Autodesk Inventor part; units mm, degrees
ref_plane "YZ Plane" through (0, 0, 0) normal (1, 0, 0) x (0, 1, 0)
ref_plane "XZ Plane" through (0, 0, 0) normal (0, 1, 0) x (-1, 0, 0)
ref_plane "XY Plane" through (0, 0, 0) normal (0, 0, 1) x (1, 0, 0)
sketch "Sketch1" plane through (0, 0, 0) normal (0, 1, 0) x (-1, 0, 0)
  circle A0 centre (0, 0) radius 6.325
  circle A1 centre (-118.053, 0) radius 6.325
  circle A2 centre (-74.04, -14.35) radius 4.5
  circle A3 centre (-74.04, 14.35) radius 4.5
  circle A4 centre (-105.29, 19.35) radius 4.5
  line L0 (-4.4447, 4.5) -> (-9.5157, 4.5)
  line L1 (-9.5157, 4.5) -> (-73.0558, 18.7411)
  line L2 (-73.329, 18.7935) -> (-104.579, 23.7935)
  line L3 (-119.775, -6.0861) -> (-75.2652, -18.68)
  line L4 (-75.2652, 18.68) -> (-119.775, 6.0861)
  line L5 (-109.79, 19.35) -> (-109.79, 8.9113)
  line L6 (-69.54, 14.35) -> (-69.54, -14.35)
  line L7 (-78.54, 14.35) -> (-78.54, -14.35)
  line L8 (-108.8889, 0) -> (-78.54, 8.5871)
  line L9 (-108.8889, 0) -> (-78.54, -8.5871)
  line L10 (-4.4447, -4.5) -> (-9.5157, -4.5)
  line L11 (-9.5157, -4.5) -> (-73.0558, -18.7411)
  line L12 (-69.54, 8.9143) -> (-29.7668, 0)
  line L13 (-29.7668, 0) -> (-69.54, -8.9143)
  line L14 (-106.001, 14.9065) -> (-74.751, 9.9065)
  line L15 (-100.79, 19.35) -> (-100.79, 11.4578)
  point P0 (-94.8865, 13.1282)
  point P1 (-100.79, 14.0728)
  dimension "d0" = 12.65
  dimension "d1" = 12.65
  dimension "d2" = 9
  dimension "d3" = 9
  dimension "d4" = 9
  dimension "d5" = 28.7
  dimension "d6" = 14.35
  dimension "d7" = 31.25
  dimension "d8" = 5
  dimension "d9" = 74.04
  dimension "d10" = 118.053
  dimension "d11" = 5.071
  dimension "d12" = 8.82
  dimension "d13" = 8.82
  dimension "d14" = 9
  dimension "d15" = 8.82
extrude "Extrusion1" add sketch "Sketch1" along normal blind 3 contours A0 | A0 L10 L11 A2 L6 L13 L12 A3 L1 L0 | A3 | A2 | L6 A2 L7 L14 A3 | A3 L4 L14 L15 A4 L2 | L3 A1 L4 L14 L7 L8 L9 A2 | L14 L7 A3 | A3 L7 L14 L4 | A4 | A1 | L15 L14 A4 | A4 L14 L15 L4 L5
sketch "Sketch2" plane through (0, 3, 0) normal (0, 1, 0) x (1, 0, 0)
  arc A0 (73.0558, -18.7411) -> (73.329, -18.7935) centre (74.04, -14.35) ccw
  circle A1 centre (74.04, -14.35) radius 4.5
  arc A2 (75.2652, 18.68) -> (73.0558, 18.7411) centre (74.04, 14.35) ccw
  arc A3 (104.579, -23.7935) -> (109.79, -19.35) centre (105.29, -19.35) ccw
  circle A4 centre (105.29, -19.35) radius 4.5
  circle A5 centre (74.04, 14.35) radius 4.5
  point P0 (0, 0)
  point P1 (109.79, -19.35)
  point P2 (73.0558, -18.7411)
  point P3 (75.2652, 18.68)
extrude "Extrusion2" add sketch "Sketch2" along normal blind 3
sketch "Sketch3" plane through (0, 3, 0) normal (0, 1, 0) x (1, 0, 0)
  arc A0 (119.775, -6.0861) -> (119.775, 6.0861) centre (118.053, 0) ccw
  circle A1 centre (118.053, 0) radius 6.325
  circle A2 centre (0, 0) radius 6.325
  arc A3 (4.4447, 4.5) -> (4.4447, -4.5) centre (0, 0) ccw
  line L0 (4.4447, -4.5) -> (18.04, -4.5)
  line L1 (18.04, -4.5) -> (18.04, 4.5)
  line L2 (18.04, 4.5) -> (4.4447, 4.5)
  line L3 (4.4447, 4.5) -> (4.4447, -4.5) construction
  point P0 (119.775, 6.0861)
  point P1 (119.775, -6.0861)
  dimension "d20" = 9
  dimension "d21" = 18.04
extrude "Extrusion3" add sketch "Sketch3" along normal blind 2
sketch "Sketch4" plane through (0, 5, 0) normal (0, 1, 0) x (1, 0, 0)
  line L0 (18.04, 4.5) -> (4.4447, 4.5)
  arc A0 (4.4447, 4.5) -> (4.4447, -4.5) centre (0, 0) ccw
  line L1 (4.4447, -4.5) -> (18.04, -4.5)
  line L2 (18.04, -4.5) -> (18.04, 4.5)
  line L3 (18.04, 4.5) -> (18.04, -4.5)
  line L4 (18.04, -4.5) -> (9.04, -4.5)
  line L5 (9.04, -4.5) -> (9.04, 4.5)
  line L6 (9.04, 4.5) -> (18.04, 4.5)
  line L7 (18.04, 4.5) -> (18.04, -4.5)
  dimension "d24" = 9
  dimension "d25" = 9
extrude "Extrusion4" add sketch "Sketch4" along normal blind 1 contours L2 L1 L5 L0
sketch "Sketch5" plane through (0, 5, 0) normal (0, 1, 0) x (1, 0, 0)
  arc A0 (4.4447, 4.5) -> (4.4447, -4.5) centre (0, 0) ccw
  circle A1 centre (118.053, 0) radius 6.325
hole "Hole1" at (0, 5, 0) at (118.053, 5, 0) direction (0, -1, 0) diameter 6 end through all
sketch "Sketch6" plane through (74.04, 6, -14.35) normal (0, 1, 0) x (1, 0, 0)
  circle A0 centre (0, 0) radius 4.5
  circle A1 centre (0, -28.7) radius 4.5
  circle A2 centre (31.25, -33.7) radius 4.5
  point P0 (-74.04, -14.35)
hole "Hole2" at (74.04, 6, -14.35) at (74.04, 6, 14.35) at (105.29, 6, 19.35) direction (0, -1, 0) diameter 4 end through all
equation "\"d0\" = d1"
equation "\"d2\" = d3"
equation "\"d3\" = d4"
equation "\"d13\" = d12"
equation "\"d15\" = d12"
properties part number "RAMPS Mount" material "ABS Plastic"
Geometry: final body of the model. Coordinates: model frame, mm. A direction names the side the tool comes from. Round coordinates to 2 decimals unless told otherwise and drop trailing zeros. Order: outer loops, then holes, each group sorted by start corner. A loop starts at its lowest first (then second) coordinate and runs counter-clockwise, first axis right, second up. Notation, with made-up numbers: (0.5, 32) -> (39.5, 32) arc R12 cw to (39.5, 50) -> close; hole circle Ø7 at (56, 61). An arc over 180 degrees is marked (long way). Use CSV: the item, a comma, the result in double quotes. Start each with the question number.
1) Set-up query: faces 4 (the face through (10, 4, 4.5)), 5 (the face through (3, 5, 1)), 6 (the face through (10, 4, -4.5)), 7 (the face through (69.54, 1, 0)), 8 (the face through (78, 3, 3)). Return all of +Z, -Z, +X, -X, +Y, -Y with unobstructed straight access to the full face (end or side cutting, diameter ignored); none if empty.
2) First-contact query: pin 1 Ø5.5 at (x, z) = (118.053, 0) entering from +Y; pin 2 Ø0.9 at (y, z) = (2, 3.5) entering from -X; pin 3 Ø3 at (x, y) = (14.5, 2.5) entering from +Z; pin 4 Ø2.5 at (y, z) = (1, 15.5) entering from +X. Flat tips, straight axial feed; report the tip coordinate or a pass-through.
3) Section D-D (x = 92). Return the cut outline in (y, z), and give its area (3 significant figures).
4) Section B-B (y = 4). State how many separate pieces and enclosed holes the cut face has, and give its area (3 significant figures).
5) Section C-C (z = -14.35). Return the cut outline in (x, y).
6) Material intervals for line 1 along Z through (x, y) = (73.5, 4.3); line 2 along Y through (x, z) = (92.5, 15.5); line 3 along Z through (x, y) = (0, 3.1) (3 decimals), sorted ascending. Write a range as from..to.
7) Draft query along Z for faces 1 (the face through (109.79, 1, 14)), 2 (the face through (74.15, 4.48, -18.85)), 3 (the face through (93.927, 1.479, -4.233)). Return one class per face: +Z half, -Z half, draft (parallel to the pull), parting line (faces both ways), or undercut.
8) Section A-A (x = 0). Return the cut outline in (y, z) (3 decimals).
Returned:
1,face 4,"+Z, +Y"
1,face 5,"+Z, -Z, -X, +Y"
1,face 6,"-Z, +Y"
1,face 7,"+Y, -Y"
1,face 8,"+Y"
2,pin 1,"passes through"
2,pin 2,"stops at x = -5.54"
2,pin 3,"stops at z = 5.95"
2,pin 4,"stops at x = 109.79"
3,outline,"(0, -13.94) -> (3, -13.94) -> (3, -4.78) -> (0, -4.78) -> close; (0, 4.78) -> (3, 4.78) -> (3, 21.78) -> (0, 21.78) -> close"
3,area,"78.5 mm²"
4,separate pieces,"5"
4,enclosed holes,"5"
4,area,"459 mm²"
5,outline,"(53.46, 0) -> (72.04, 0) -> (72.04, 6) -> (69.54, 6) -> (69.54, 3) -> (53.46, 3) -> close; (76.04, 0) -> (90.57, 0) -> (90.57, 3) -> (78.54, 3) -> (78.54, 6) -> (76.04, 6) -> close"
6,line 1,"z = -18.82..-16.28, -12.42..-9.88, 9.88..12.42, 16.28..18.82"
6,line 2,"y = 0..3"
6,line 3,"z = -6.325..-3, 3..6.325"
7,face 1,"draft"
7,face 2,"-Z half"
7,face 3,"undercut"
8,outline,"(0, -6.325) -> (5, -6.325) -> (5, -3) -> (0, -3) -> close; (0, 3) -> (5, 3) -> (5, 6.325) -> (0, 6.325) -> close"
